from build123d import *

# Parameters (mm, degrees)
CROQUIS3_W              = 35
CROQUIS3_H              = 25
SALIENTE_EXTRUIR1_DEPTH = 3
CROQUIS4_R              = 12.5
SALIENTE_EXTRUIR2_DEPTH = 15
REDONDEO1_R             = 12.5


with BuildPart() as part:
    # Croquis3 → Saliente-Extruir1 (new body)
    with BuildSketch(Plane(origin=(0, 0, 0), x_dir=(1, 0, 0), z_dir=(0, 1, 0))):
        Rectangle(CROQUIS3_W, CROQUIS3_H)
    extrude(amount=SALIENTE_EXTRUIR1_DEPTH)

    # Croquis4 → Saliente-Extruir2 (add)
    with BuildSketch(Plane(origin=(0, 3, 0), x_dir=(1, 0, 0), z_dir=(0, 1, 0))):
        with Locations(Location((0, 0, 0), (0, 0, 270))):
            Circle(CROQUIS4_R)
    extrude(amount=SALIENTE_EXTRUIR2_DEPTH)

    # Redondeo1
    redondeo1_edges = [part.edges().sort_by_distance(p)[0] for p in [
        (0, 18, -12.5),
    ]]
    fillet(redondeo1_edges, radius=REDONDEO1_R)


solid = part.part
Source: CAD feature listing. Evaluate the final solid. Frame: model axes, mm. A direction names the side the tool comes from. Round coordinates to 2 decimals unless told otherwise and drop trailing zeros. Loops run counter-clockwise (first coordinate to the right, second up) from the corner with the lowest first, then second, coordinate; pieces in that order, holes last. Notation, with made-up numbers: (37.5, -5) - (83.5, -5) arc R9 ccw to (83.5, 11) - close; hole circle Ø9 at (50.25, -25.75). An arc over 180 degrees is marked (long way). Write item = value, one per line. Start each with the question number.
(1) Ray query, line 1 along Y through (x, z) = (15.5, 4.25); line 2 along Z through (x, y) = (-5.5, 8); line 3 along X through (y, z) = (5.5, -10.75). Return the intervals inside material, ascending. Write a range as from..to.
(2) Section query C-C, the plane y = 16.5. Output: boundary loops of the cut face in (x, z), plus the area to 3 significant figures.
(3) Section query A-A, the plane x = -12. Output: boundary loops of the cut face in (y, z).
(4) Section query D-D, the plane y = 11.25. Output: boundary loops of the cut face in (x, z).
(5) Section query B-B, the plane z = 0. Output: boundary loops of the cut face in (x, y).
(6) Set-up query: faces 1 (the face through (3.755, 4.232, 11.923)), 2 (the face through (0, 0, 0)). Return all of +Z, -Z, +X, -X, +Y, -Y with unobstructed straight access to the full face (end or side cutting, diameter ignored); none if empty.
(7) Pin query (flat end, axial travel): pin 1 (1 mm diameter, centred on x = -6.5, y = 9, fed in from -Z); pin 2 (6 mm diameter, centred on y = 13, z = 1, fed in from +X); pin 3 (8 mm diameter, centred on y = 10, z = 1, fed in from -X). Return the tip coordinate at first contact, or that it passes through.
Conclusion:
q1.line_1 = 0..3
q1.line_2 = -10.94..10.94
q1.line_3 = -6.38..6.38
q2.outline = circle Ø11.87 at (0, 0)
q2.area = 111 mm2
q3.outline = (0, -12.5) - (3, -12.5) - (3, -3.5) - (5.5, -3.5) arc R3.5 ccw to (5.5, 3.5) - (3, 3.5) - (3, 12.5) - (0, 12.5) - close
q4.outline = circle Ø22.2 at (0, 0)
q5.outline = (-17.5, 0) - (17.5, 0) - (17.5, 3) - (12.5, 3) - (12.5, 5.5) arc R12.5 ccw to (-12.5, 5.5) - (-12.5, 3) - (-17.5, 3) - close
q6.face_1 = +Y
q6.face_2 = +Z, -Z, +X, -X, -Y
q7.pin_1 = -10.43
q7.pin_2 = 11.64
q7.pin_3 = -12.49
